Autodesk Inventor part; units mm, degrees
ref_plane "YZ Plane" through (0, 0, 0) normal (1, 0, 0) x (0, 1, 0)
ref_plane "XZ Plane" through (0, 0, 0) normal (0, 1, 0) x (-1, 0, 0)
ref_plane "XY Plane" through (0, 0, 0) normal (0, 0, 1) x (1, 0, 0)
sketch "Sketch1" plane through (0, 0, 0) normal (0, 1, 0) x (-1, 0, 0)
  circle A0 centre (0, 0) radius 30
  dimension "d0" = 60
extrude "Extrusion1" add sketch "Sketch1" along normal blind 10
sketch "Sketch2" plane through (0, 10, 0) normal (0, 1, 0) x (1, 0, 0)
  circle A0 centre (0, 0) radius 14.245
  dimension "d3" = 28.49
extrude "Extrusion2" add sketch "Sketch2" along normal blind 5
sketch "Sketch3" plane through (0, 10, 0) normal (0, 1, 0) x (1, 0, 0)
  circle A0 centre (-25.3377, 0) radius 1.27
  point P0 (0, 0)
  dimension "d6" = 2.54
  dimension "d7" = 25.3377
extrude "Extrusion3" cut sketch "Sketch3" against normal up to surface (10 mm away)
sketch "Sketch4" plane through (0, 15, 0) normal (0, 1, 0) x (1, 0, 0)
  circle A0 centre (0, 0) radius 2.1
  dimension "d10" = 4.2
extrude "Extrusion4" cut sketch "Sketch4" against normal up to surface (15 mm away)
chamfer "Chamfer1" distance 1 angle 45 1 edges at (-14.245, 15, 0)
sketch "Sketch6" plane through (0, 10, 0) normal (0, 1, 0) x (1, 0, 0)
  circle A0 centre (-25.3377, 0) radius 1.27
  circle A1 centre (-25.3377, 0) radius 1.27
  line L0 (-25.3377, 0) -> (0, 0) construction
  line L1 (0, 0) -> (-24.0976, 7.8298) construction
  circle A2 centre (0, 0) radius 25.3377 construction
  circle A3 centre (-24.0976, 7.8298) radius 1.27
  circle A4 centre (-24.0976, -7.8298) radius 1.27
  circle A5 centre (-14.8931, -20.4986) radius 1.27
  circle A6 centre (0, -25.3377) radius 1.27
  circle A7 centre (14.8931, -20.4986) radius 1.27
  circle A8 centre (24.0976, -7.8298) radius 1.27
  circle A9 centre (24.0976, 7.8298) radius 1.27
  circle A10 centre (14.8931, 20.4986) radius 1.27
  circle A11 centre (0, 25.3377) radius 1.27
  circle A12 centre (-14.8931, 20.4986) radius 1.27
  point P0 (-24.9704, -1.2157)
  point P1 (-24.9704, 1.2157)
  dimension "d22" = 18
  dimension "d23" = 2.54
  dimension "d24" = 2.54
  dimension "d27" = 360
extrude "Extrusion6" cut sketch "Sketch6" against normal up to surface (10 mm away) contours A3 | A4 | A5 | A6 | A7 | A8 | A9 | A10 | A11 | A12
sketch "Sketch7" plane through (0, 10, 0) normal (0, 1, 0) x (1, 0, 0)
  circle A0 centre (0, 0) radius 14.245
  circle A1 centre (0, 0) radius 16.245
  dimension "d31" = 2
extrude "Extrusion7" add sketch "Sketch7" along normal blind 1.5
sketch "Sketch8" plane through (0, 10, 0) normal (0, 1, 0) x (1, 0, 0)
  circle A0 centre (0, 0) radius 16.245
  circle A1 centre (0, -25.3377) radius 1.27
  circle A2 centre (-24.0976, -7.8298) radius 1.27
  circle A3 centre (-14.8931, 20.4986) radius 1.27
  circle A4 centre (24.0976, -7.8298) radius 1.27
  circle A5 centre (24.0976, 7.8298) radius 1.27
  circle A6 centre (-24.0976, 7.8298) radius 1.27
  circle A7 centre (-14.8931, -20.4986) radius 1.27
  circle A8 centre (0, 25.3377) radius 1.27
  circle A9 centre (14.8931, -20.4986) radius 1.27
  circle A10 centre (14.8931, 20.4986) radius 1.27
  circle A11 centre (-25.3377, 0) radius 1.27
  circle A12 centre (0, 0) radius 30
  circle A13 centre (0, 0) radius 16.245
  circle A14 centre (0, 0) radius 14.245
equation "\"d24\" = d23"
properties part number "bottom"
Source: CAD feature listing. Evaluate the final solid. Frame: model axes, mm. A direction names the side the tool comes from. Round coordinates to 2 decimals unless told otherwise and drop trailing zeros. Loops run counter-clockwise (first coordinate to the right, second up) from the corner with the lowest first, then second, coordinate; pieces in that order, holes last.
Q1. Section C-C, the plane y = 13. Return loops of the section in (x, z) (3 decimals), plus the area to 3 significant figures.
Q2. Section D-D, the plane y = 6. State how many separate pieces and enclosed holes the cut face has, plus the area to 3 significant figures.
Q3. Ray query, line 1 (Z direction, x = 0, y = 3.5); line 2 (Z direction, x = -14.5, y = 1.5); line 3 (Y direction, x = -24.5, z = 4.5). Return the intervals inside material, ascending.
Q4. Section A-A, the plane x = 0. Return loops of the section in (y, z) (3 decimals).
Q5. Section B-B, the plane z = 0. Return loops of the section in (x, y) (3 decimals).
Q6. First-contact query: P1, Ø4, axis at y = 10, z = 23.5, coming from the -X side; P2, Ø3.5, axis at x = -14.89, z = -20.5, coming from the +Y side; P3, Ø2, axis at x = 24.1, z = -7.83, coming from the +Y side; P4, Ø3, axis at x = -24.1, z = 7.83, coming from the -Y side. Flat tips, straight axial feed; report the tip coordinate or a pass-through.
Q7. Mould query, pull axis X, two halves, no side actions, for faces 3 (the face through (13.159, 12.732, -5.456)), 4 (the face through (-22.886, 5.07, 7.448)), 5 (the face through (-0.1, 11.5, 14.4)). Classes: pulls with the +X half, pulls with the -X half, needs draft (parallel to the pull), parting line crosses it, or undercut.
Q8. Access query for faces 1 (the face through (0, 0, -6)), 2 (the face through (-13, 10, -13)). Directions: +Z, -Z, +X, -X, +Y, -Y. A direction counts if a zero-diameter tool reaches every point of the face in a straight line with its end or side. Return the directions, or none.
Solutions:
1. outline: circle Ø28.49 at (0, 0); hole circle Ø4.2 at (0, 0)
1. area: 624 mm2
2. separate pieces: 1
2. enclosed holes: 12
2. area: 2,760 mm2
3. line 1: z = -30 to -26.61, -24.07 to -2.1, 2.1 to 24.07, 26.61 to 30
3. line 2: z = -26.26 to -21.71, -19.29 to 19.29, 21.71 to 26.26
3. line 3: y = 0 to 10
4. outline: (0, -30) - (10, -30) - (10, -26.608) - (0, -26.608) - close; (0, -24.068) - (10, -24.068) - (10, -16.245) - (11.5, -16.245) - (11.5, -14.245) - (14, -14.245) - (15, -13.245) - (15, -2.1) - (0, -2.1) - close; (0, 2.1) - (15, 2.1) - (15, 13.245) - (14, 14.245) - (11.5, 14.245) - (11.5, 16.245) - (10, 16.245) - (10, 24.068) - (0, 24.068) - close; (0, 26.608) - (10, 26.608) - (10, 30) - (0, 30) - close
5. outline: (-30, 0) - (-26.608, 0) - (-26.608, 10) - (-30, 10) - close; (-24.068, 0) - (-2.1, 0) - (-2.1, 15) - (-13.245, 15) - (-14.245, 14) - (-14.245, 11.5) - (-16.245, 11.5) - (-16.245, 10) - (-24.068, 10) - close; (2.1, 0) - (30, 0) - (30, 10) - (16.245, 10) - (16.245, 11.5) - (14.245, 11.5) - (14.245, 14) - (13.245, 15) - (2.1, 15) - close
6. P1: stops at x = -20.92
6. P2: stops at y = 10
6. P3: passes through
6. P4: stops at y = 0
7. face 3: parting line crosses it
7. face 4: undercut
7. face 5: needs draft
8. face 1: +Z, -Z, +X, -X, -Y
8. face 2: +Y
